Job drawing, mm, ordinate dimensions from the low corner. One solid piece. A direction names the side the tool comes from. Round coordinates to 2 decimals unless told otherwise and drop trailing zeros. Loops run counter-clockwise (first coordinate to the right, second up) from the corner with the lowest first, then second, coordinate; pieces in that order, holes last. Notation, with made-up numbers: M 42.25,-22.75 L 82.25,-22.75 A4 ccw 82.25,-15.75 Z; hole C -22.75,13 d3. An arc over 180 degrees is marked long. Use one line per item in the form item = value. Start each with the question number.
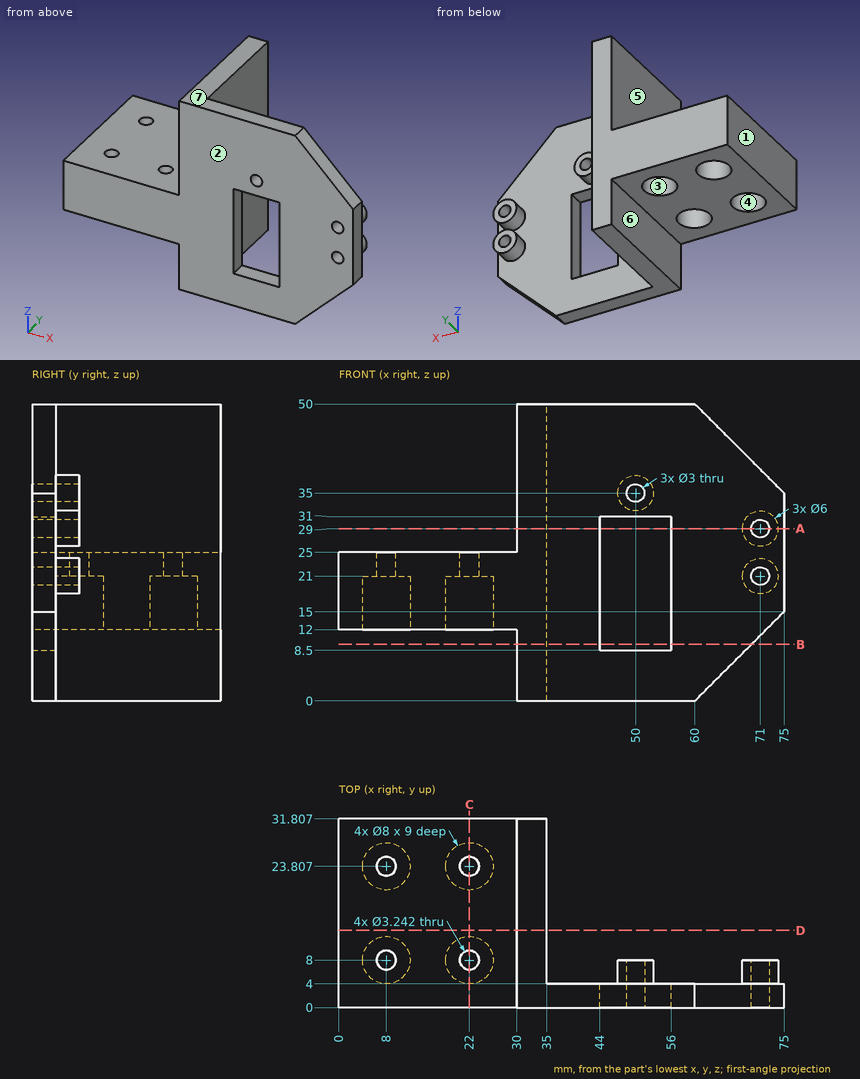
Q1. Drop flat-ended pins along their axis: P1, Ø4, axis at x = 60, z = 21.5, coming from the -Y side; P2, Ø9, axis at x = 6.5, y = 9.5, coming from the -Z side; P3, Ø8.5, axis at y = 12.5, z = 16, coming from the +X side; P4, Ø2.5, axis at x = 24, y = 9.5, coming from the -Z side. Give the stop position or say it passes through.
Q2. Wall check: probe 1 along Z at (x, y) = (71, 6.25); probe 2 along Y at (x, z) = (22, 24); probe 3 along X at (y, z) = (23, 16). Give the ranges that are in metal, low to high.
Q3. Saw through at D-D (y = 13). Give the cut face in (x, z), and give its area (3 significant figures).
Q4. Pull direction X, two halves, no side cores. Call the marked faces 1, 2 and 3: pulls with the +X half, pulls with the -X half, needs draft (parallel to the pull), parting line crosses it, or undercut.
Q5. Tool access for the marked faces 4, 5, 6 and 7: list every direction of +Z, -Z, +X, -X, +Y, -Y with a clear straight run to the whole face (end or side of a thin tool).
Q6. Saw through at B-B (z = 9.5). Give the cut face in (x, y).
Q7. Saw through at A-A (z = 29). Give the cut face in (x, y).
Q8. Saw through at C-C (x = 22). Give the cut face in (y, z), and give its area (3 significant figures).
Filled in:
q1.P1 = 0
q1.P2 = 12
q1.P3 = 35
q1.P4 = 21
q2.probe_1 = 18 to 19.5, 22.5 to 24, 26 to 27.5, 30.5 to 32
q2.probe_2 = 0 to 6.38, 9.62 to 22.19, 25.43 to 31.81
q2.probe_3 = 0 to 4.08, 11.92 to 18.08, 25.92 to 35
q3.outline = M 0,12 L 30,12 L 30,0 L 35,0 L 35,50 L 30,50 L 30,25 L 0,25 Z
q3.area = 640 mm²
q4.face_1 = pulls with the -X half
q4.face_2 = needs draft
q4.face_3 = undercut
q5.face_4 = -Z
q5.face_5 = +Z, -X, +Y, -Y
q5.face_6 = -Z, -X, +Y, -Y
q5.face_7 = +Z, +X, -X, +Y, -Y
q6.outline = M 30,0 L 44,0 L 44,4 L 35,4 L 35,31.81 L 30,31.81 Z; M 56,0 L 69.5,0 L 69.5,4 L 56,4 Z
q7.outline = M 30,0 L 44,0 L 44,4 L 35,4 L 35,31.81 L 30,31.81 Z; M 56,0 L 69.5,0 L 69.5,8 L 68,8 L 68,4 L 56,4 Z; M 72.5,0 L 75,0 L 75,4 L 74,4 L 74,8 L 72.5,8 Z
q8.outline = M 0,12 L 4,12 L 4,21 L 6.38,21 L 6.38,25 L 0,25 Z; M 9.62,21 L 12,21 L 12,12 L 19.81,12 L 19.81,21 L 22.19,21 L 22.19,25 L 9.62,25 Z; M 25.43,21 L 27.81,21 L 27.81,12 L 31.81,12 L 31.81,25 L 25.43,25 Z
q8.area = 244 mm²
